Source: CAD feature listing. Evaluate the final solid. Frame: model axes, mm. Round coordinates to 2 decimals unless told otherwise and drop trailing zeros. Loops run counter-clockwise (first coordinate to the right, second up) from the corner with the lowest first, then second, coordinate; pieces in that order, holes last. Notation, with made-up numbers: (57, 74) -> (111, 74) arc R18 cw to (111, 85) -> close; hole circle Ø8 at (-7, 46.5). An arc over 180 degrees is marked (long way). Put each result on its own line as item: value. Start each with the question number.
1. Material intervals for L1, parallel to X at y = 14.5, z = 506.5; L2, parallel to X at y = 4, z = 288.5, sorted ascending.
2. Cut plane B-B (y = 8). Return the cut outline in (x, z).
3. Contact query for flat-ended pins moving along their axis: pin 1 (10 mm diameter, centred on x = 15, y = 11, fed in from -Z); pin 2 (1.5 mm diameter, centred on y = 15, z = 303, fed in from +X); pin 3 (1 mm diameter, centred on x = 8.5, z = 94.5, fed in from +Y). Output: stop coordinate, or through.
```python
from build123d import *

# Parameters (mm, degrees)
F1_DEPTH = 558.8


with BuildPart() as f1:
    # F0 (on Top) → F1 (new body)
    with BuildSketch(Plane.XY):
        with BuildLine():
            Line((0, 19.05), (0, 0))
            Line((0, 0), (19.05, 0))
            Line((19.05, 0), (19.05, 1.0795))
            ThreePointArc((19.05, 1.0795), (18.90121, 1.43871), (18.542, 1.5875))
            Line((18.542, 1.5875), (4.7625, 1.5875))
            ThreePointArc((4.7625, 1.5875), (2.517436, 2.517436), (1.5875, 4.7625))
            Line((1.5875, 4.7625), (1.5875, 18.542))
            ThreePointArc((1.5875, 18.542), (1.43871, 18.90121), (1.0795, 19.05))
            Line((1.0795, 19.05), (0, 19.05))
        make_face()
    extrude(amount=F1_DEPTH)


solid = f1.part
```
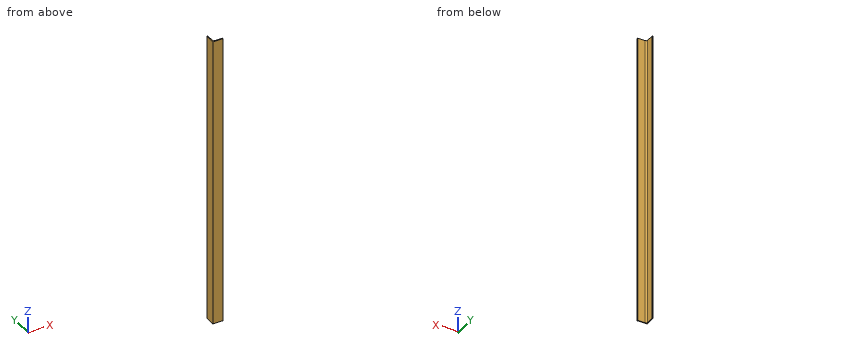
Solution:
1. L1: x = 0 to 1.59
1. L2: x = 0 to 1.68
2. outline: (0, 0) -> (1.59, 0) -> (1.59, 558.8) -> (0, 558.8) -> close
3. pin 1: passes through
3. pin 2: stops at x = 1.59
3. pin 3: stops at y = 1.59
